```python
from build123d import *

# Parameters (mm, degrees)
PAD_DEPTH               = 40
POCKET_DEPTH            = 36.001
SKETCH002_R             = 1
PAD001_DEPTH            = 8
SKETCH002_MIRRORED_2_R  = 1
PAD001_MIRRORED_2_DEPTH = 8
POCKET001_DEPTH         = 41.001
POCKET002_DEPTH         = 5


with BuildPart() as part:
    # Sketch → Pad (new body)
    with BuildSketch(Plane.XY.offset(-4)):
        with BuildLine():
            Line((-35, 31), (35, 31))
            ThreePointArc((41, 25), (39.242641, 29.242641), (35, 31))
            Line((41, 25), (41, -25))
            ThreePointArc((35, -31), (39.242641, -29.242641), (41, -25))
            Line((35, -31), (-35, -31))
            ThreePointArc((-41, -25), (-39.242641, -29.242641), (-35, -31))
            Line((-41, -25), (-41, 25))
            ThreePointArc((-35, 31), (-39.242641, 29.242641), (-41, 25))
        make_face()
    extrude(amount=PAD_DEPTH)

    # Sketch001 → Pocket (cut, through all)
    with BuildSketch(Plane.XY):
        with BuildLine():
            Line((-31, 23), (31, 23))
            ThreePointArc((33, 21), (32.414214, 22.414214), (31, 23))
            Line((33, 21), (33, -21))
            ThreePointArc((31, -23), (32.414214, -22.414214), (33, -21))
            Line((31, -23), (-31, -23))
            ThreePointArc((-33, -21), (-32.414214, -22.414214), (-31, -23))
            Line((-33, -21), (-33, 21))
            ThreePointArc((-31, 23), (-32.414214, 22.414214), (-33, 21))
        make_face()
    extrude(amount=POCKET_DEPTH, mode=Mode.SUBTRACT)

    # Sketch002 → Pad001 (join)
    with BuildSketch(Plane.XY):
        with BuildLine():
            Line((-30, 20), (-25, 20))
            ThreePointArc((-30, 15), (-26.464466, 16.464466), (-25, 20))
            Line((-30, 20), (-30, 15))
        make_face()
        with Locations((-28, 18)):
            Circle(SKETCH002_R, mode=Mode.SUBTRACT)
    pad001 = extrude(amount=PAD001_DEPTH)

    # Sketch002 Mirrored 2 → Pad001 Mirrored 2 (add)
    with BuildSketch(Plane(origin=(0, 0, 0), x_dir=(-1, 0, 0), z_dir=(0, 0, -1))):
        with BuildLine():
            Line((-30, 20), (-25, 20))
            ThreePointArc((-30, 15), (-26.464466, 16.464466), (-25, 20))
            Line((-30, 20), (-30, 15))
        make_face()
        with Locations((-28, 18)):
            Circle(SKETCH002_MIRRORED_2_R, mode=Mode.SUBTRACT)
    pad001_mirrored_2 = extrude(amount=-PAD001_MIRRORED_2_DEPTH)

    # Mirrored001: Pad001, Pad001 Mirrored 2 across Sketch002 H_Axis
    add(pad001.mirror(Plane.ZX))
    add(pad001_mirrored_2.mirror(Plane.ZX))

    # Sketch003 → Pocket001 (cut, through all)
    with BuildSketch(Plane.YZ):
        with BuildLine():
            Line((0, 20), (-10, 20))
            ThreePointArc((-12, 22), (-11.414214, 20.585786), (-10, 20))
            Line((-12, 22), (-12, 27))
            ThreePointArc((-10, 29), (-11.414214, 28.414214), (-12, 27))
            Line((-10, 29), (0, 29))
            ThreePointArc((2, 27), (1.414214, 28.414214), (0, 29))
            Line((2, 27), (2, 22))
            ThreePointArc((0, 20), (1.414214, 20.585786), (2, 22))
        make_face()
    extrude(amount=POCKET001_DEPTH, mode=Mode.SUBTRACT)

    # Sketch004 (on Face7 of Pocket001) → Pocket002 (cut)
    with BuildSketch(Plane(origin=(0, 31, 0), x_dir=(-1, 0, 0), z_dir=(0, 1, 0))):
        with BuildLine():
            Line((-22, 25), (-14, 25))
            ThreePointArc((-12, 23), (-12.585786, 24.414214), (-14, 25))
            Line((-12, 23), (-12, 10))
            Line((-12, 10), (-24, 10))
            Line((-24, 10), (-24, 23))
            ThreePointArc((-22, 25), (-23.414214, 24.414214), (-24, 23))
        make_face()
        with BuildLine():
            Line((2, 16), (13, 16))
            ThreePointArc((15, 14), (14.414214, 15.414214), (13, 16))
            Line((15, 14), (15, 10))
            Line((15, 10), (0, 10))
            Line((0, 10), (0, 14))
            ThreePointArc((2, 16), (0.585786, 15.414214), (0, 14))
        make_face()
    extrude(amount=-POCKET002_DEPTH, mode=Mode.SUBTRACT)


solid = part.part
```
Work out the finished part from the listing and answer in its coordinate system (mm). A direction names the side the tool comes from. Coordinates: 2 decimals unless noted, no trailing zeros. Order: outer loops, then holes, each group sorted by start corner. A loop starts at its lowest first (then second) coordinate and runs counter-clockwise, first axis right, second up. Notation, with made-up numbers: M 73,-37 L 97,-37 A13 cw 97,-30 Z; hole C -5,53 d1. An arc over 180 degrees is marked long. Use CSV: the item, a comma, the result in double quotes.
1) For faces 1 (the face through (1, -27, 36)), 2 (the face through (36.94, 1.43, 28.4)), 3 (the face through (41, 0, 16)), 4 (the face through (24, 29, 16)), 5 (the face through (-33, 0, 18)), determine the directions among +Z, -Z, +X, -X, +Y, -Y from which every point of the face is accessible in a straight line to the end or side of a thin tool.
Worked out:
face 1,"+Z, +X, -X, +Y, -Y"
face 2,"+X"
face 3,"+Z, -Z, +X, +Y, -Y"
face 4,"+Y"
face 5,"+Z"
2) Section C-C on z = 30.5 is taken. Write down the section's boundary in (x, y).
Worked out:
outline,"M -41,-25 A6 ccw -35,-31 L 35,-31 A6 ccw 41,-25 L 41,25 A6 ccw 35,31 L -35,31 A6 ccw -41,25 Z; hole M -33,-21 A2 ccw -31,-23 L 31,-23 A2 ccw 33,-21 L 33,21 A2 ccw 31,23 L -31,23 A2 ccw -33,21 Z"
3) Section B-B on y = -1 is taken. Write down the section's boundary in (x, z), plus the area to 3 significant figures.
Worked out:
outline,"M -41,-4 L 41,-4 L 41,20 L 33,20 L 33,0 L -33,0 L -33,36 L -41,36 Z; M 33,29 L 41,29 L 41,36 L 33,36 Z"
area,"832 mm^2"
4) Determine the mould class of faces 6 (the face through (39.289, 29.196, 15.72)), 7 (the face through (23.4, 28.54, 24.43)), 8 (the face through (-28, -20, 4)) for opening direction Y: released by +Y, released by -Y, zero draft, split by the parting line, or undercut.
Worked out:
face 6,"released by +Y"
face 7,"zero draft"
face 8,"undercut"
5) Consider line 1 (X direction, y = 20, z = 26.5); line 2 (Y direction, x = -11.5, z = 13); line 3 (Y direction, x = 4, z = 15.5). Determine where each line is inside the solid, lowest interval first. Write a range as [from, to].
Worked out:
line 1,"x = [-41, -33], [33, 41]"
line 2,"y = [-31, -23], [23, 26]"
line 3,"y = [-31, -23], [23, 31]"
6) Section D-D on x = -8.5 is taken. Write down the section's boundary in (y, z).
Worked out:
outline,"M -31,-4 L 31,-4 L 31,10 L 26,10 L 26,16 L 31,16 L 31,36 L 23,36 L 23,0 L -23,0 L -23,36 L -31,36 Z"
7) Flat-ended cylindrical pins translate along their axes: pin 1 Ø2.5 at (x, y) = (-26.5, 17) entering from +Z; pin 2 Ø4 at (y, z) = (27.5, 18.5) entering from +X; pin 3 Ø1.2 at (y, z) = (29.5, 11) entering from -X. Find the tip coordinate at first contact, or state that the pin passes through.
Worked out:
pin 1,"stops at z = 8"
pin 2,"stops at x = 40.98"
pin 3,"stops at x = -39.56"
8) Section A-A on z = 1 is taken. Count the separate pieces of the cut face and the enclosed holes in it, plus the area to 3 significant figures.
Worked out:
separate pieces,"5"
enclosed holes,"5"
area,"2,090 mm^2"
